Check sheet for the modelled part. Datum: model origin and axes. Units: mm. A direction names the side the tool comes from. Give positions to 0.01 mm unless a question says otherwise; leave off trailing zeros. Order: outer loops, then holes, each group sorted by start corner. A loop starts at its lowest first (then second) coordinate and runs counter-clockwise, first axis right, second up. Notation, with made-up numbers: (29.25, 77.5) -> (41.25, 77.5) arc R35 ccw to (41.25, 110.5) -> close; hole circle Ø1 at (62, 21.5). An arc over 180 degrees is marked (long way). One line per question, with ' | ' between items.
```python
from build123d import *

# Parameters (mm, degrees)
SKETCH2_R          = 2.54
CUT_EXTRUDE1_DEPTH = 30.003356194
SHELL2_T           = -0.254


with BuildPart() as part:
    # Sketch1 → Revolve1 (revolve)
    with BuildSketch(Plane.XY, mode=Mode.PRIVATE) as revolve1_sk:
        Polygon((0, 0), (0, 17.224827156), (15.25, 17.224827156), (15.25, 8.612413578), (16.5, 8.612413578), (16.5, 0), align=None)
    revolve(revolve1_sk.sketch.rotate(Axis((0, 0, 0), (0, 1, 0)), 90), axis=Axis((0, 0, 0), (0, 1, 0)))

    # Sketch2 → Cut-Extrude1 (cut, through all)
    with BuildSketch(Plane(origin=(0, 17.224827156, 0), x_dir=(1, 0, 0), z_dir=(0, 1, 0))):
        with Locations(Location((0, 0, 0), (0, 0, 270))):
            Circle(SKETCH2_R)
    extrude(amount=-CUT_EXTRUDE1_DEPTH, mode=Mode.SUBTRACT)

    # Shell2
    shell2_openings = [part.faces().sort_by_distance(p)[0] for p in [
        (0, 0, 16.033309524),
    ]]
    offset(amount=SHELL2_T, openings=shell2_openings, kind=Kind.INTERSECTION)


solid = part.part
```
Q1. Thickness scan on line 1 (X direction, y = 13, z = 0); line 2 (X direction, y = 5.5, z = 0); line 3 (Z direction, x = 2, y = 8). Record the ranges inside material, lowest first.
Result sheet:
line 1: x = -15.25 to -15, -2.79 to -2.54, 2.54 to 2.79, 15 to 15.25 | line 2: x = -16.5 to -16.25, -2.79 to -2.54, 2.54 to 2.79, 16.25 to 16.5 | line 3: z = -16.38 to -16.12, -1.95 to -1.57, 1.57 to 1.95, 16.12 to 16.38
Q2. Section check A-A (z = 0). Enter the section's corners in (x, y).
Result sheet:
outline: (-16.5, 0) -> (-16.25, 0) -> (-16.25, 8.36) -> (-15, 8.36) -> (-15, 16.97) -> (-2.79, 16.97) -> (-2.79, 0) -> (-2.54, 0) -> (-2.54, 17.22) -> (-15.25, 17.22) -> (-15.25, 8.61) -> (-16.5, 8.61) -> close; (2.54, 0) -> (2.79, 0) -> (2.79, 16.97) -> (15, 16.97) -> (15, 8.36) -> (16.25, 8.36) -> (16.25, 0) -> (16.5, 0) -> (16.5, 8.61) -> (15.25, 8.61) -> (15.25, 17.22) -> (2.54, 17.22) -> close
Q3. Section check D-D (z = 14.5). Enter the section's corners in (x, y).
Result sheet:
outline: (-7.87, 0) -> (-7.33, 0) -> (-7.33, 8.36) -> (-3.82, 8.36) -> (-3.82, 16.97) -> (3.82, 16.97) -> (3.82, 8.36) -> (7.33, 8.36) -> (7.33, 0) -> (7.87, 0) -> (7.87, 8.61) -> (4.72, 8.61) -> (4.72, 17.22) -> (-4.72, 17.22) -> (-4.72, 8.61) -> (-7.87, 8.61) -> close
Q4. Section check C-C (y = 9.75). Enter the section's corners in (x, z).
Result sheet:
outline: circle Ø30.5 at (0, 0); circle Ø5.59 at (0, 0); hole circle Ø29.99 at (0, 0); hole circle Ø5.08 at (0, 0)
Q5. Access from +Z, -Z, +X, -X, +Y, -Y to the whole of each face (thin tool, end or side, straight path). Record for faces 4 (the face through (-4.956, 4.246, -15.738)), 5 (the face through (15.86, 4.12, 3.52)).
Result sheet:
face 4: +Y, -Y | face 5: -Y
Q6. Section check B-B (x = 0). Enter the section's corners in (y, z), and give its area (3 significant figures).
Result sheet:
outline: (0, -16.5) -> (8.61, -16.5) -> (8.61, -15.25) -> (17.22, -15.25) -> (17.22, -2.54) -> (0, -2.54) -> (0, -2.79) -> (16.97, -2.79) -> (16.97, -15) -> (8.36, -15) -> (8.36, -16.25) -> (0, -16.25) -> close; (0, 2.54) -> (17.22, 2.54) -> (17.22, 15.25) -> (8.61, 15.25) -> (8.61, 16.5) -> (0, 16.5) -> (0, 16.25) -> (8.36, 16.25) -> (8.36, 15) -> (16.97, 15) -> (16.97, 2.79) -> (0, 2.79) -> close | area: 24.3 mm2
Q7. Depth check by flat-ended pin: pin 1 Ø1.5 at (y, z) = (11.5, 1) entering from +X; pin 2 Ø1 at (x, y) = (-11.5, 13) entering from -Z; pin 3 Ø5 at (y, z) = (10, 2.5) entering from -X. Enter the tip coordinate at first touch or a pass-through.
Result sheet:
pin 1: stops at x = 15.25 | pin 2: stops at z = -10.56 | pin 3: stops at x = -16.49
Q8. Mould release check, pull along Z, two halves, no side actions. Record for faces 1 (the face through (5, 8.612, 15)), 2 (the face through (14.887, 12.858, 3.306)), 3 (the face through (2.52, 8.73, -0.33)): pulls with the +Z half, pulls with the -Z half, needs draft (parallel to the pull), parting line crosses it, or undercut.
Result sheet:
face 1: needs draft | face 2: parting line crosses it | face 3: undercut
